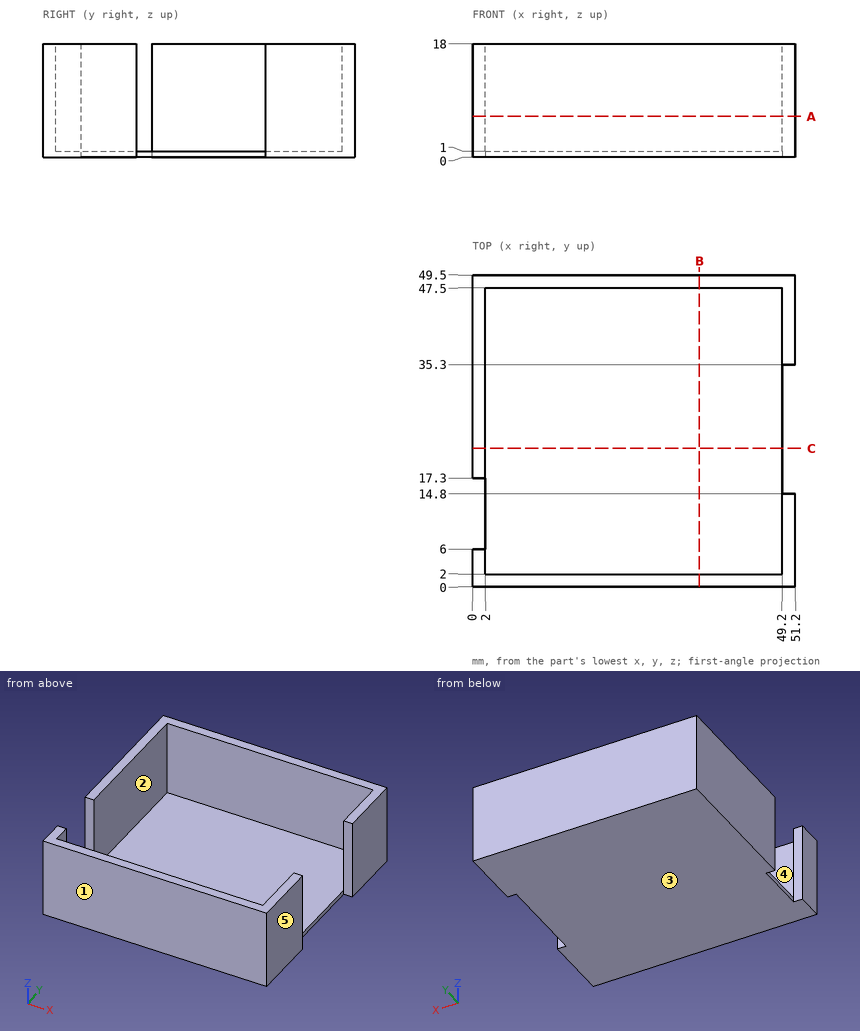
The drawing under review shows one solid part. Ordinate dimensions are in mm from its lowest x, y, z. A direction names the side the tool comes from. Round coordinates to 2 decimals unless told otherwise and drop trailing zeros. Loops run counter-clockwise (first coordinate to the right, second up) from the corner with the lowest first, then second, coordinate; pieces in that order, holes last. Notation, with made-up numbers: (-27, 42.25) - (-2, 42.25) arc R20 ccw to (-2, 60.25) - close; hole circle Ø11 at (53.5, 7.5). An arc over 180 degrees is marked (long way). One line per question, with ' | ' between items.
Q1. The part is to be moulded in two halves that separate along Y. For the marked faces 1, 2 and 3, say which applies: released by +Y, released by -Y, zero draft, split by the parting line, or undercut.
Taken from the geometry:
face 1: released by -Y | face 2: undercut | face 3: zero draft
Q2. For line 1 along X through (y, z) = (44, 5); line 2 along Y through (x, z) = (18, 8.5); line 3 along X through (y, z) = (23, 10.75), list the stretches that pass through material, from the lowest coordinate up. Write a range as [from, to].
Taken from the geometry:
line 1: x = [0, 2], [49.2, 51.2] | line 2: y = [0, 2], [47.5, 49.5] | line 3: x = [0, 2]
Q3. Tool access review of the marked faces 4 and 5: name each direction out of +Z, -Z, +X, -X, +Y, -Y from which nothing blocks a thin tool from reaching the whole face with its end or side.
Taken from the geometry:
face 4: +Z | face 5: +Z, -Z, +X, +Y, -Y
Q4. Take a section at A-A (z = 6.5). Give the boundary of the cut face in (x, y).
Taken from the geometry:
outline: (0, 0) - (51.2, 0) - (51.2, 14.8) - (49.2, 14.8) - (49.2, 2) - (2, 2) - (2, 6) - (0, 6) - close; (0, 17.3) - (2, 17.3) - (2, 47.5) - (49.2, 47.5) - (49.2, 35.3) - (51.2, 35.3) - (51.2, 49.5) - (0, 49.5) - close
Q5. For pin 1 (4 mm diameter, centred on x = 26.5, y = 42.5, fed in from -Z); pin 2 (6 mm diameter, centred on y = 26, z = 9, fed in from +X); pin 3 (12 mm diameter, centred on x = 13.5, y = 11.5, fed in from +Z); pin 4 (0.8 mm diameter, centred on y = 14.5, z = 0.5, fed in from -X), all flat-tipped, find the tip position at first contact; note any pin that passes through.
Taken from the geometry:
pin 1: stops at z = 0 | pin 2: stops at x = 2 | pin 3: stops at z = 1 | pin 4: stops at x = 2
Q6. Take a section at C-C (y = 22). Give the boundary of the cut face in (x, z), and give its area (3 significant figures).
Taken from the geometry:
outline: (0, 0) - (49.2, 0) - (49.2, 1) - (2, 1) - (2, 18) - (0, 18) - close | area: 83.2 mm²
Q7. Take a section at B-B (x = 36). Give the boundary of the cut face in (y, z).
Taken from the geometry:
outline: (0, 0) - (49.5, 0) - (49.5, 18) - (47.5, 18) - (47.5, 1) - (2, 1) - (2, 18) - (0, 18) - close
